Autodesk Inventor part; units mm, degrees
ref_plane "YZ Plane" through (0, 0, 0) normal (1, 0, 0) x (0, 1, 0)
ref_plane "XZ Plane" through (0, 0, 0) normal (0, 1, 0) x (-1, 0, 0)
ref_plane "XY Plane" through (0, 0, 0) normal (0, 0, 1) x (1, 0, 0)
sketch "Sketch1" plane through (0, 0, 0) normal (0, 1, 0) x (-1, 0, 0)
  line L0 (0, 0) -> (60, 0)
  line L1 (60, 0) -> (60, -63)
  line L2 (60, -63) -> (0, -63)
  line L3 (0, -63) -> (0, 0)
  dimension "d0" = 60
  dimension "d1" = 63
extrude "Extrusion1" add sketch "Sketch1" along normal blind 8
sketch "Esboço2" plane through (0, 8, 0) normal (0, 1, 0) x (1, 0, 0)
  line L0 (0, 63) -> (-60, 63)
  line L1 (-60, 63) -> (-60, 0)
  line L2 (-60, 0) -> (0, 0)
  point P0 (-37.5, 36)
  point P1 (-22.5, 36)
  point P2 (-22.5, 26)
  point P3 (-37.5, 26)
  dimension "d5" = 0
  dimension "d6" = 15
  dimension "d7" = 0
  dimension "d8" = 15
  dimension "d9" = 10
  dimension "d10" = 0
  dimension "d11" = 60
  dimension "d12" = 22.5
  dimension "d20" = 26
hole "Furo1" at (-37.5, 8, -36) at (-22.5, 8, -36) at (-22.5, 8, -26) at (-37.5, 8, -26) direction (0, -1, 0) diameter 3.242 depth 8
sketch "Sketch3" plane through (0, 0, -63) normal (0, 0, -1) x (-1, 0, 0)
  point P0 (0, 0)
sketch "Sketch4" plane through (0, 0, 0) normal (1, 0, 0) x (0, 0, -1)
  line L0 (63, 0) -> (63, 8)
  line L1 (0, 0) -> (0, 8)
  point P0 (55.0003, 4.0635)
  point P1 (8, 4.0565)
  point P2 (63, 4)
  point P3 (0, 4)
  dimension "d21" = 8
  dimension "d22" = 8
hole "Hole2" at (0, 4.0635, -55.0003) at (0, 4.0565, -8) direction (-1, 0, 0) diameter 4.134 depth 14.2 tip angle 118
sketch "Sketch5" plane through (-60, 0, -63) normal (-1, 0, 0) x (0, 0, 1)
  circle A0 centre (55, 4.0565) radius 2.067
  circle A1 centre (7.9997, 4.0635) radius 2.067
  point P0 (63, 0)
hole "Hole3" at (-60, 4.0565, -8) at (-60, 4.0635, -55.0003) direction (1, 0, 0) diameter 4.134 depth 14.2 tip angle 118
equation "\"d18\" = Thickness"
equation "\"BendRadius\" = Thickness"
equation "\"BendReliefWidth\" = Thickness"
equation "\"BendReliefDepth\" = 0.5 * Thickness"
equation "\"CornerReliefSize\" = 4 * Thickness"
equation "\"MinimumRemnant\" = 2 * Thickness"
equation "\"TransitionRadius\" = BendRadius"
equation "\"JacobiRadiusSize\" = BendRadius"
equation "\"GapSize\" = Thickness"
properties part number "Frente da caixa de susentação" material "Aluminum 6061"
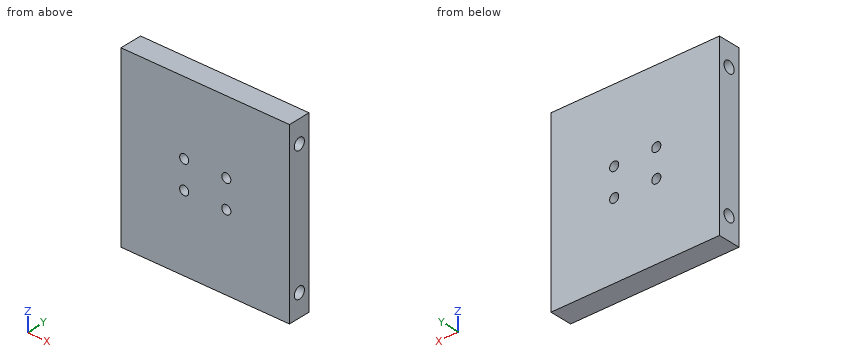
Work out the finished part from the listing and answer in its coordinate system (mm). Round coordinates to 2 decimals unless told otherwise and drop trailing zeros. Loops run counter-clockwise (first coordinate to the right, second up) from the corner with the lowest first, then second, coordinate; pieces in that order, holes last.
(1) Each of these flat-tipped pins is pushed along its axis until it touches: P1, Ø8, axis at x = -16.5, z = -27.5, coming from the -Y side; P2, Ø3.5, axis at y = 4.06, z = -55, coming from the -X side. Where does it stop, or does it pass through?
Computed values:
P1: stops at y = 0
P2: stops at x = -45.61
(2) The part is cut by section C-C, the plane y = 3. Give the number of separate pieces and of enclosed holes in the cut face, and give its area (3 significant figures).
Computed values:
separate pieces: 1
enclosed holes: 4
area: 3,540 mm2
(3) The part is cut by section B-B, the plane z = -26. Give the vertices of the cut face in (x, y), and give its area (3 significant figures).
Computed values:
outline: (-60, 0) - (-39.12, 0) - (-39.12, 8) - (-60, 8) - close; (-35.88, 0) - (-24.12, 0) - (-24.12, 8) - (-35.88, 8) - close; (-20.88, 0) - (0, 0) - (0, 8) - (-20.88, 8) - close
area: 428 mm2
(4) Find the intervals of material crossed by L1, parallel to X at y = 3.25, z = -36; L2, parallel to Z at x = -37.5, y = 6; L3, parallel to Z at x = -38, y = 5.75, in increasing order.
Computed values:
L1: x = -60 to -39.12, -35.88 to -24.12, -20.88 to 0
L2: z = -63 to -37.62, -34.38 to -27.62, -24.38 to 0
L3: z = -63 to -37.54, -34.46 to -27.54, -24.46 to 0
(5) The part is cut by section A-A, the plane x = -22.5. Give the vertices of the cut face in (y, z), and give its area (3 significant figures).
Computed values:
outline: (0, -63) - (8, -63) - (8, -37.62) - (0, -37.62) - close; (0, -34.38) - (8, -34.38) - (8, -27.62) - (0, -27.62) - close; (0, -24.38) - (8, -24.38) - (8, 0) - (0, 0) - close
area: 452 mm2
